The listing builds one solid part. Answer for the finished solid, in the listing's coordinates (mm). Round coordinates to 2 decimals unless told otherwise and drop trailing zeros. Order: outer loops, then holes, each group sorted by start corner. A loop starts at its lowest first (then second) coordinate and runs counter-clockwise, first axis right, second up. Notation, with made-up numbers: (-31.75, -24) -> (18.25, -24) arc R20 cw to (18.25, -18) -> close; hole circle Ø5 at (-5.75, -13). An arc over 180 degrees is marked (long way). Return JSON: item names as keys, results as strings. Group by question number.
(1) Consider line 1 (X direction, y = 3.1, z = 298); line 2 (Z direction, x = 206, y = 4.35); line 3 (Z direction, x = 287, y = 0.6). Determine where each line is inside the solid, lowest interval first. Write a range as [from, to].
(2) The part is cut by section A-A (x = 28.5). Determine the outline of the cut face in (y, z).
(3) The part is cut by section C-C (y = 2). Count the separate pieces of the cut face and the enclosed holes in it, plus the area to 3 significant figures.
(4) The part is cut by section B-B (z = 265.5). Determine the outline of the cut face in (x, y).
(5) Each of these flat-tipped pins is pushed along its axis until it touches: pin 1 (2.5 mm diameter, centred on y = 2.5, z = 282.5, fed in from -X); pin 2 (2.5 mm diameter, centred on y = 3.5, z = -13.5, fed in from -X). Where does it stop, or does it pass through?
from build123d import *

# Parameters (mm, degrees)
SKETCH1_W           = 400
SKETCH1_H           = 400
BOSS_EXTRUDE1_DEPTH = 5
SKETCH2_W           = 120
SKETCH2_H           = 50
SKETCH2_W_2         = 50
SKETCH2_H_2         = 120
CUT_EXTRUDE1_DEPTH  = 5
SKETCH4_R           = 2
SKETCH4_R_2         = 1.5
CUT_EXTRUDE2_DEPTH  = 5


with BuildPart() as part:
    # Sketch1 → Boss-Extrude1 (new body)
    with BuildSketch(Plane(origin=(0, 0, 0), x_dir=(1, 0, 0), z_dir=(0, 1, 0))):
        with Locations((163.492063492, -170.952380952)):
            Rectangle(SKETCH1_W, SKETCH1_H)
    extrude(amount=BOSS_EXTRUDE1_DEPTH)

    # Sketch2 → Cut-Extrude1 (cut)
    with BuildSketch(Plane(origin=(0, 5, 0), x_dir=(1, 0, 0), z_dir=(0, 1, 0))):
        with Locations((23.492063492, 4.047619048)):
            Rectangle(SKETCH2_W, SKETCH2_H)
        with Locations((338.492063492, -30.952380952)):
            Rectangle(SKETCH2_W_2, SKETCH2_H_2)
        with Locations((303.492063492, -345.952380952)):
            Rectangle(SKETCH2_W, SKETCH2_H)
        with Locations((-11.507936508, -310.952380952)):
            Rectangle(SKETCH2_W_2, SKETCH2_H_2)
    extrude(amount=-CUT_EXTRUDE1_DEPTH, mode=Mode.SUBTRACT)

    # Sketch4 → Cut-Extrude2 (cut)
    with BuildSketch(Plane(origin=(0, 5, 0), x_dir=(1, 0, 0), z_dir=(0, 1, 0))):
        with Locations(Location((284.092063492, -212.952380952, 0), (0, 0, 270))):
            Circle(SKETCH4_R)
        with Locations(Location((275.092063492, -212.952380952, 0), (0, 0, 270))):
            Circle(SKETCH4_R)
        with Locations(Location((284.092063492, 21.047619048, 0), (0, 0, 270))):
            Circle(SKETCH4_R)
        with Locations(Location((275.092063492, 21.047619048, 0), (0, 0, 270))):
            Circle(SKETCH4_R)
        with Locations(Location((286.292063492, -13.552380952, 0), (0, 0, 270))):
            Circle(SKETCH4_R_2)
        with Locations(Location((274.292063492, -13.552380952, 0), (0, 0, 270))):
            Circle(SKETCH4_R_2)
        with Locations(Location((286.292063492, -43.352380952, 0), (0, 0, 270))):
            Circle(SKETCH4_R_2)
        with Locations(Location((274.292063492, -43.352380952, 0), (0, 0, 270))):
            Circle(SKETCH4_R_2)
        with Locations(Location((355.492063492, -291.552380952, 0), (0, 0, 270))):
            Circle(SKETCH4_R)
        with Locations(Location((355.492063492, -282.552380952, 0), (0, 0, 270))):
            Circle(SKETCH4_R)
        with Locations(Location((320.892063492, -293.752380952, 0), (0, 0, 270))):
            Circle(SKETCH4_R_2)
        with Locations(Location((320.892063492, -281.752380952, 0), (0, 0, 270))):
            Circle(SKETCH4_R_2)
        with Locations(Location((291.092063492, -293.752380952, 0), (0, 0, 270))):
            Circle(SKETCH4_R_2)
        with Locations(Location((291.092063492, -281.752380952, 0), (0, 0, 270))):
            Circle(SKETCH4_R_2)
        with Locations(Location((121.492063492, -291.552380952, 0), (0, 0, 270))):
            Circle(SKETCH4_R)
        with Locations(Location((121.492063492, -282.552380952, 0), (0, 0, 270))):
            Circle(SKETCH4_R)
        with Locations(Location((51.892063492, -362.952380952, 0), (0, 0, 270))):
            Circle(SKETCH4_R)
        with Locations(Location((42.892063492, -362.952380952, 0), (0, 0, 270))):
            Circle(SKETCH4_R)
        with Locations(Location((52.692063492, -328.352380952, 0), (0, 0, 270))):
            Circle(SKETCH4_R_2)
        with Locations(Location((40.692063492, -328.352380952, 0), (0, 0, 270))):
            Circle(SKETCH4_R_2)
        with Locations(Location((52.692063492, -298.552380952, 0), (0, 0, 270))):
            Circle(SKETCH4_R_2)
        with Locations(Location((40.692063492, -298.552380952, 0), (0, 0, 270))):
            Circle(SKETCH4_R_2)
        with Locations(Location((51.892063492, -128.952380952, 0), (0, 0, 270))):
            Circle(SKETCH4_R)
        with Locations(Location((42.892063492, -128.952380952, 0), (0, 0, 270))):
            Circle(SKETCH4_R)
        with Locations(Location((-28.507936508, -59.352380952, 0), (0, 0, 270))):
            Circle(SKETCH4_R)
        with Locations(Location((-28.507936508, -50.352380952, 0), (0, 0, 270))):
            Circle(SKETCH4_R)
        with Locations(Location((35.892063492, -60.152380952, 0), (0, 0, 270))):
            Circle(SKETCH4_R_2)
        with Locations(Location((35.892063492, -48.152380952, 0), (0, 0, 270))):
            Circle(SKETCH4_R_2)
        with Locations(Location((6.092063492, -60.152380952, 0), (0, 0, 270))):
            Circle(SKETCH4_R_2)
        with Locations(Location((6.092063492, -48.152380952, 0), (0, 0, 270))):
            Circle(SKETCH4_R_2)
        with Locations(Location((205.492063492, -59.352380952, 0), (0, 0, 270))):
            Circle(SKETCH4_R)
        with Locations(Location((205.492063492, -50.352380952, 0), (0, 0, 270))):
            Circle(SKETCH4_R)
    extrude(amount=-CUT_EXTRUDE2_DEPTH, mode=Mode.SUBTRACT)


solid = part.part
Answer below:
{
 "1": {"line 1": "x = [13.49, 39.3], [42.09, 51.3], [54.09, 363.49]", "line 2": "z = [-29.05, 48.42], [52.29, 57.42], [61.29, 370.95]", "line 3": "z = [-29.05, 12.23], [14.87, 42.03], [44.67, 320.95]"},
 "2": {"outline": "(0, 20.95) -> (5, 20.95) -> (5, 370.95) -> (0, 370.95) -> close"},
 "3": {"separate pieces": "1", "enclosed holes": "32", "area": "136,000 mm²"},
 "4": {"outline": "(13.49, 0) -> (363.49, 0) -> (363.49, 5) -> (13.49, 5) -> close"},
 "5": {"pin 1": "stops at x = 13.49", "pin 2": "stops at x = 83.49"}
}
